```python
from build123d import *

# Parameters (mm, degrees)
SKETCH1_R           = 2.25
BOSS_EXTRUDE1_DEPTH = 12.7
FILLET1_R           = 12.7
FILLET2_R           = 6.35
FILLET3_R           = 1


with BuildPart() as part:
    # Sketch1 → Boss-Extrude1 (new body)
    # profile 1 of 2: a face of its own
    with BuildSketch(Plane(origin=(0, 0, 0), x_dir=(0, 0, -1), z_dir=(1, 0, 0))):
        Polygon((48.592196898, 40.156684656), (39.611940777, 49.136940777), (-6.35, 3.175), (-6.35, -31.75), (6.35, -31.75), (6.35, -2.085512242), align=None)
        with Locations((0, -25.4)):
            Circle(SKETCH1_R, mode=Mode.SUBTRACT)
        Circle(SKETCH1_R, mode=Mode.SUBTRACT)
    # profile 2 of 2: a face of its own
    with BuildSketch(Plane(origin=(0, 0, 0), x_dir=(0, 0, -1), z_dir=(1, 0, 0))):
        Polygon((54.079029807, 24.430314129), (48.592196898, 40.156684656), (39.611940777, 31.176428535), align=None)
    extrude(amount=BOSS_EXTRUDE1_DEPTH)

    # Fillet1
    fillet1_edges = [part.edges().sort_by_distance(p)[0] for p in [
        (6.35, 3.175, 6.35),
        (6.35, 49.136940777, -39.611940777),
    ]]
    fillet(fillet1_edges, radius=FILLET1_R - 0.0001)  # a hair under: the kernel refuses the full size

    # Fillet2
    fillet2_edges = [part.edges().sort_by_distance(p)[0] for p in [
        (6.35, 31.176428535, -39.611940777),
        (6.35, -2.085512242, -6.35),
    ]]
    fillet(fillet2_edges, radius=FILLET2_R)
    fillet2_2_edges = [part.edges().sort_by_distance(p)[0] for p in [
        (6.35, 40.156684656, -48.592196898),
        (6.35, -31.75, 6.35),
        (6.35, -31.75, -6.35),
    ]]
    fillet(fillet2_2_edges, radius=FILLET2_R - 0.0004)  # a hair under: the kernel refuses the full size

    # Fillet3
    fillet3_edges = [part.edges().sort_by_distance(p)[0] for p in [
        (0, 26.863823768, -48.860351546),
        (6.35, 24.430314129, -54.079029807),
        (0, -13.74293541, 6.35),
        (12.7, -13.74293541, 6.35),
        (0, 23.525734978, -14.000734978),
        (0, 43.818086311, -38.395583818),
        (0, 2.774570502, 5.383277675),
        (12.7, 23.525734978, -14.000734978),
        (12.7, 2.774570502, 5.383277675),
        (12.7, 43.818086311, -38.395583818),
        (0, 31.48135692, -51.618964812),
        (0, 13.903383358, -22.338895601),
        (12.7, 26.863823768, -48.860351546),
        (0, -15.058084182, -6.35),
        (0, -29.890245218, -4.490245218),
        (0, -29.890245218, 4.490245218),
        (0, 40.316018936, -48.193567347),
        (12.7, 31.48135692, -51.618964812),
        (12.7, -15.058084182, -6.35),
        (12.7, 13.903383358, -22.338895601),
        (12.7, -29.890245218, -4.490245218),
        (12.7, -29.890245218, 4.490245218),
        (12.7, 40.316018936, -48.193567347),
        (0, 29.795808191, -39.855381394),
        (12.7, 29.795808191, -39.855381394),
        (0, -2.285728568, -6.833364969),
        (12.7, -2.285728568, -6.833364969),
    ]]
    fillet(fillet3_edges, radius=FILLET3_R)


solid = part.part
```
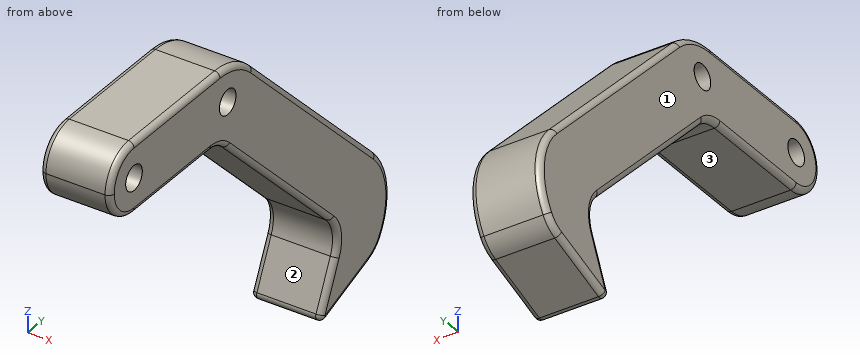
Geometry: final body of the model. Coordinates: model frame, mm. Face numbers are marked on the shaded views. Round coordinates to 2 decimals unless told otherwise and drop trailing zeros. Order: outer loops, then holes, each group sorted by start corner. A loop starts at its lowest first (then second) coordinate and runs counter-clockwise, first axis right, second up. Notation, with made-up numbers: M 10.5,6 L 37.5,6 A12 cw 37.5,10 Z; hole C -17,38 d7. An arc over 180 degrees is marked long. One line per item, written item: value.
(1) Pin query (flat end, axial travel): P1, Ø1, axis at x = 10.5, z = -15.5, coming from the -Y side; P2, Ø4, axis at y = 0, z = 0, coming from the -X side; P3, Ø1.5, axis at x = 9.5, z = -41, coming from the +Y side; P4, Ø5, axis at x = 3, y = -15.5, coming from the -Z side. Return the tip coordinate at first contact, or that it passes through.
Result sheet:
P1: y = 6.56
P2: through
P3: y = 43.86
P4: z = -6.35
(2) Line query: probe 1 along Y at (x, z) = (7.5, 0) (3 decimals); probe 2 along Z at (x, y) = (8.75, 28) (3 decimals); probe 3 along Z at (x, y) = (4, -24.5). Output: solid intervals per line, ascending. Write a range as [from, to].
Result sheet:
probe 1: [-31.75, -27.65], [-23.15, -2.25], [2.25, 9.525]
probe 2: [-52.834, -46.424], [-36.436, -18.475]
probe 3: [-6.35, -2.06], [2.06, 6.35]
(3) Cut plane B-B (x = 6.75). Give the number of separate pieces and of enclosed holes in the cut face, and give its area (3 significant figures).
Result sheet:
separate pieces: 1
enclosed holes: 2
area: 1,210 mm2
(4) Pull-direction query (Z, two-part tool) for the marked faces 1, 2 and 3; classes: pulls with the +Z half, pulls with the -Z half, needs draft (parallel to the pull), parting line crosses it, or undercut.
Result sheet:
face 1: needs draft
face 2: undercut
face 3: pulls with the -Z half
(5) Cut plane A-A (y = -21). Return the cut outline in (x, z), and give its area (3 significant figures).
Result sheet:
outline: M 0,-5.35 A1 ccw 1,-6.35 L 11.7,-6.35 A1 ccw 12.7,-5.35 L 12.7,5.35 A1 ccw 11.7,6.35 L 1,6.35 A1 ccw 0,5.35 Z
area: 160 mm2
